from build123d import *

# Parameters (mm, degrees)
F0_R     = 17
F1_DEPTH = 10
F2_R     = 21
F3_DEPTH = 25
F3_TAPER = 10
F4_R     = 3


with BuildPart() as f1:
    # F0 (on Top) → F1 (new body)
    with BuildSketch(Plane.XY):
        Circle(F0_R)
    extrude(amount=F1_DEPTH)

    # F2 (on face) → F3 (join)
    with BuildSketch(Plane.XY.offset(10)):
        Circle(F2_R)
    extrude(amount=F3_DEPTH, taper=F3_TAPER)

    # F4
    f4_edges = [f1.edges().sort_by_distance(p)[0] for p in [
        (-16.591825, 0, 35),
        (-17, 0, 0),
    ]]
    fillet(f4_edges, radius=F4_R)


solid = f1.part
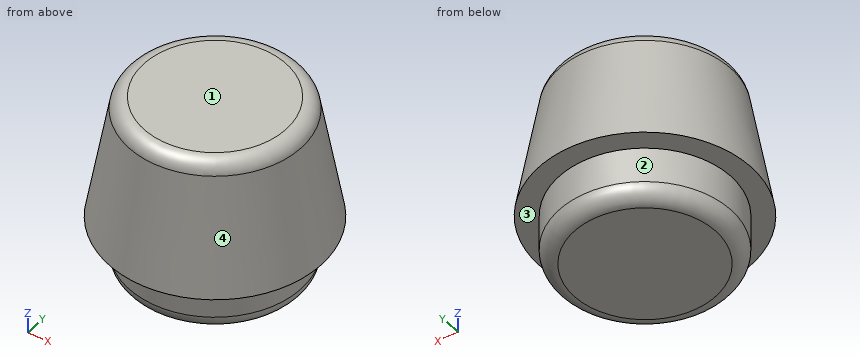
Design review of the part built by this model. Coordinates are the model's own, in mm. Face numbers are marked on the shaded views. A direction names the side the tool comes from. Give positions to 0.01 mm unless a question says otherwise; leave off trailing zeros. Write each loop counter-clockwise with the first axis right and the second up, starting at its lowest first coordinate (ties: lowest second). Pieces come first, ordered by that corner, then holes. Notation, with made-up numbers: M 60,-33.75 L 94,-33.75 A21 cw 94,-8.75 Z; hole C -24.5,22.25 d6. An arc over 180 degrees is marked long. Answer as a JSON object with one key per item and string values. Group by question number.
1) Clearance check with flat-ended pins moving along their axes: pin 1 Ø1.5 at (x, z) = (0.5, 18.5) entering from +Y; pin 2 Ø3 at (x, y) = (-14.5, -11) entering from +Z; pin 3 Ø1 at (x, z) = (-13.5, 26.5) entering from -Y. State where each tip first meets the part, or that it passes through.
2) We need section C-C (z = 13.5). Give the boundary of the cut face in (x, y).
3) For line 1 along X through (y, z) = (-5.5, 26.5); line 2 along X through (y, z) = (13.5, 18); line 3 along Y through (x, z) = (16, 26), list the stretches that pass through material, from the lowest coordinate up.
4) We need section A-A (y = 0). Give the boundary of the cut face in (x, z).
5) We need section D-D (z = 22.5). Give the boundary of the cut face in (x, y), and give its area (3 significant figures).
6) Tool access review of the marked faces 1 and 2: name each direction out of +Z, -Z, +X, -X, +Y, -Y from which nothing blocks a thin tool from reaching the whole face with its end or side.
7) Mouldability with a two-part tool opening along Y and no side actions: class the marked faces 3 and 4 as released by +Y, released by -Y, zero draft, split by the parting line, or undercut.
Answer key:
{
 "1": {"pin 1": "stops at y = 19.63", "pin 2": "stops at z = 33.45", "pin 3": "stops at y = -12.6"},
 "2": {"outline": "C 0,0 d40.77"},
 "3": {"line 1": "x = -17.23 to 17.23", "line 2": "x = -14.19 to 14.19", "line 3": "y = -8.63 to 8.63"},
 "4": {"outline": "M -21,10 L -17,10 L -17,3 A3 ccw -14,0 L 14,0 A3 ccw 17,3 L 17,10 L 21,10 L 17.03,32.52 A3 ccw 14.07,35 L -14.07,35 A3 ccw -17.03,32.52 Z"},
 "5": {"outline": "C 0,0 d37.59", "area": "1,110 mm²"},
 "6": {"face 1": "+Z, +X, -X, +Y, -Y", "face 2": "-Z"},
 "7": {"face 3": "zero draft", "face 4": "split by the parting line"}
}
